Autodesk Inventor part; units mm, degrees
ref_plane "YZ Plane" through (0, 0, 0) normal (1, 0, 0) x (0, 1, 0)
ref_plane "XZ Plane" through (0, 0, 0) normal (0, 1, 0) x (-1, 0, 0)
ref_plane "XY Plane" through (0, 0, 0) normal (0, 0, 1) x (1, 0, 0)
sketch "Sketch1" plane through (0, 0, 0) normal (0, 0, 1) x (1, 0, 0)
  line L0 (0, 0) -> (127, 0) construction
  line L1 (0, 0) -> (63.5, 0) construction
  line L2 (63.5, 0) -> (63.5, 25.4) construction
  line L3 (0, 0) -> (0, 1.7272)
  line L4 (127, 0) -> (127, 1.7272)
  line L5 (63.5, 25.4) -> (63.5, 27.1272)
  line L6 (63.5, 25.4) -> (65.2272, 25.4) construction
  arc A0 (127, 1.7272) -> (0, 1.7272) centre (63.5, -64.9478) ccw
  line L7 (38.1, 21.8272) -> (88.9, 21.8272)
  arc A1 (127, 0) -> (88.9, 21.8272) centre (63.5, -66.675) ccw
  arc A2 (38.1, 21.8272) -> (0, 0) centre (63.5, -66.675) ccw
  dimension "d0" = 127
  dimension "d1" = 63.5
  dimension "d2" = 25.4
  dimension "d3" = 1.7272
  dimension "d4" = 1.7272
  dimension "d5" = 1.7272
  dimension "d6" = 90
  dimension "d8" = 50.8
extrude "Extrusion1" add sketch "Sketch1" along normal blind 12.7
properties part number "ClipBottom"
For this review, take the finished solid that the model builds, in its own axes (mm). A direction names the side the tool comes from. Round coordinates to 2 decimals unless told otherwise and drop trailing zeros. Loops run counter-clockwise (first coordinate to the right, second up) from the corner with the lowest first, then second, coordinate; pieces in that order, holes last. Notation, with made-up numbers: (38.25, -13.75) - (69.25, -13.75) arc R19 cw to (69.25, 6.25) - close; hole circle Ø11 at (54.5, 78.5). An arc over 180 degrees is marked (long way). Put each result on its own line as item: value. Start each with the question number.
1. For faces 1 (the cylindrical face through (109, 13.37, 6.26)), 2 (the flat face through (63, 23, 0)), list the 3-axis set-ups (+Z, -Z, +X, -X, +Y, -Y) from which the entire face can be reached by the end or side of a thin tool; tool diameter is ignored.
2. Consider section B-B on z = 1.25. State the section outline as (x, y) points (3 decimals).
3. Insertion check: P1, Ø6, axis at x = 15.5, z = 6.5, coming from the -Y side; P2, Ø1, axis at y = 13.5, z = 9, coming from the +X side; P3, Ø4, axis at y = 9.5, z = 9.5, coming from the +X side. Each pin has a flat end and moves straight along its axis. Give the tip position at first contact, or say it passes through.
4. Consider section A-A on y = 6.5. State the section outline as (x, z) points.
5. Consider section D-D on x = 113. State the section outline as (y, z) points.
6. Consider section C-C on x = 41.5. State the section outline as (y, z) points.
7. For probe 1 along X at (y, z) = (2, 5.25); probe 2 along X at (y, z) = (9, 2); probe 3 along Y at (x, z) = (102, 11.5), list the stretches that pass through material, from the lowest coordinate up. Write a range as [from, to].
8. Mouldability with a two-part tool opening along X and no side actions: class faces 3 (the cylindrical face through (62.52, 27.12, 6.26)), 4 (the cylindrical face through (17.461, 13.063, 6.261)), 5 (the flat face through (63, 21.827, 6)), 6 (the flat face through (63, 23, 12.7)) as +X half, -X half, draft (parallel to the pull), parting line (faces both ways), or undercut.
Result sheet:
1. face 1: +Z, -Z, -Y
1. face 2: -Z, +X, -X, +Y, -Y
2. outline: (0, 0) arc R92.076 cw to (38.1, 21.827) - (88.9, 21.827) arc R92.074 cw to (127, 0) - (127, 1.727) arc R92.075 ccw to (0, 1.727) - close
3. P1: y = 9.99
3. P2: x = 112.51
3. P3: x = 120.33
4. outline: (5.42, 0) - (7.61, 0) - (7.61, 12.7) - (5.42, 12.7) - close; (119.39, 0) - (121.58, 0) - (121.58, 12.7) - (119.39, 12.7) - close
5. outline: (10.96, 0) - (12.69, 0) - (12.69, 12.7) - (10.96, 12.7) - close
6. outline: (21.83, 0) - (24.46, 0) - (24.46, 12.7) - (21.83, 12.7) - close
7. probe 1: [0.29, 2.17], [124.83, 126.71]
7. probe 2: [8.64, 11.05], [115.95, 118.36]
7. probe 3: [16.96, 18.69]
8. face 3: parting line
8. face 4: undercut
8. face 5: undercut
8. face 6: draft
